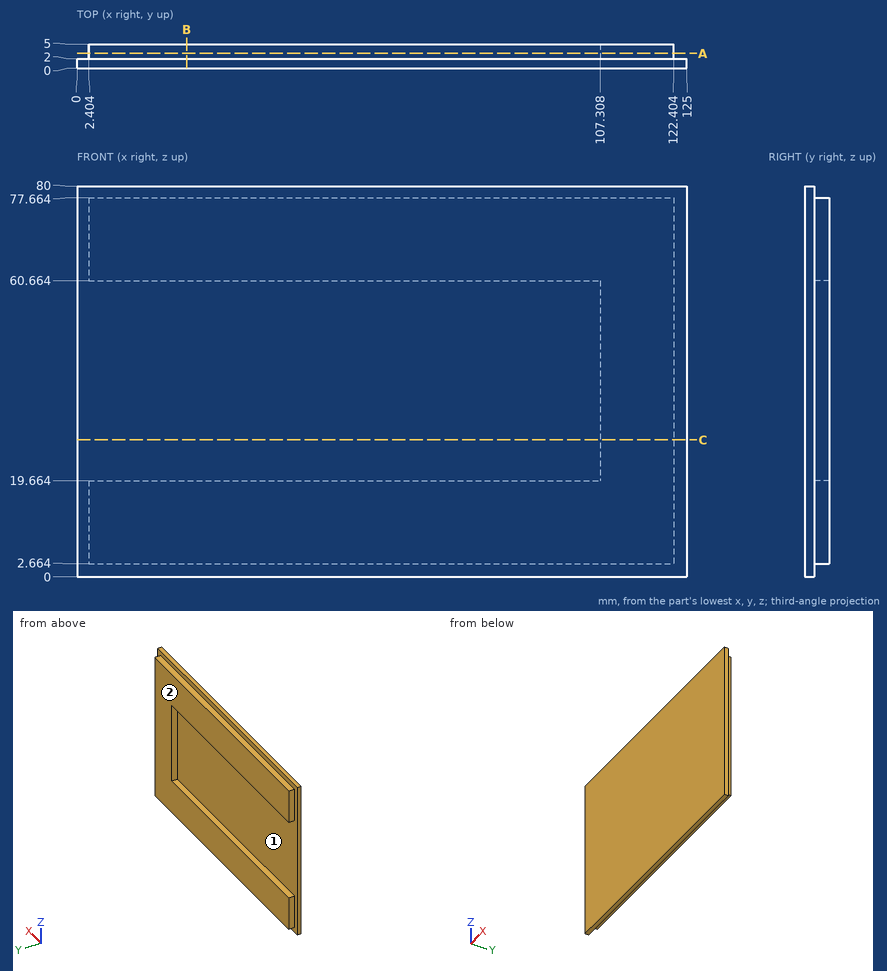
Drawing for the job (mm, zero at the part's lowest x, y, z). Round coordinates to 2 decimals unless told otherwise and drop trailing zeros. Loops run counter-clockwise (first coordinate to the right, second up) from the corner with the lowest first, then second, coordinate; pieces in that order, holes last.
1. Band-saw the part on A-A, the plane y = 3.1. List the corners of the cut face in (x, z).
Check values:
outline: (2.4, 2.66) - (122.4, 2.66) - (122.4, 77.66) - (2.4, 77.66) - (2.4, 60.66) - (107.31, 60.66) - (107.31, 19.66) - (2.4, 19.66) - close
2. Wall check: probe 1 along Z at (x, y) = (30.5, 2.6); probe 2 along X at (y, z) = (2.2, 59); probe 3 along Z at (x, y) = (115, 3.05). Give the ranges that are in metal, low to high.
Check values:
probe 1: z = 2.66 to 19.66, 60.66 to 77.66
probe 2: x = 107.31 to 122.4
probe 3: z = 2.66 to 77.66
3. Band-saw the part on B-B, the plane x = 22.5. List the corners of the cut face in (y, z).
Check values:
outline: (0, 0) - (2, 0) - (2, 2.66) - (5, 2.66) - (5, 19.66) - (2, 19.66) - (2, 60.66) - (5, 60.66) - (5, 77.66) - (2, 77.66) - (2, 80) - (0, 80) - close
4. Band-saw the part on C-C, the plane z = 28. List the corners of the cut face in (x, y).
Check values:
outline: (0, 0) - (125, 0) - (125, 2) - (122.4, 2) - (122.4, 5) - (107.31, 5) - (107.31, 2) - (0, 2) - close
5. Drop flat-ended pins along their axis: P1, Ø1.5, axis at y = 4, z = 20.5, coming from the +X side; P2, Ø3, axis at x = 67, y = 4, coming from the +Z side; P3, Ø0.9, axis at y = 3.5, z = 73.5, coming from the -X side. Give the stop position or say it passes through.
Check values:
P1: stops at x = 122.4
P2: stops at z = 77.66
P3: stops at x = 2.4
6. Mould opens along Z. For the marked faces 1 and 2 say: +Z half, -Z half, draft (parallel to the pull), parting line (faces both ways), or undercut.
Check values:
face 1: undercut
face 2: draft
